Here's how the part is built. I have some questions about the finished solid (model axes, mm). A direction names the side the tool comes from. Give positions to 0.01 mm unless a question says otherwise; leave off trailing zeros. Order: outer loops, then holes, each group sorted by start corner. A loop starts at its lowest first (then second) coordinate and runs counter-clockwise, first axis right, second up. Notation, with made-up numbers: M 57.5,35.5 L 101.5,35.5 A16 cw 101.5,52.5 Z; hole C 44,-6 d8. An arc over 180 degrees is marked long. Use one line per item in the form item = value.
from build123d import *

# Parameters (mm, degrees)
SKETCH1_R           = 14
BOSS_EXTRUDE1_DEPTH = 19
BOSS_EXTRUDE2_DEPTH = 0.8128
SKETCH3_R           = 2.1
CUT_EXTRUDE1_DEPTH  = 0.8128
SKETCH4_R           = 4.5
BOSS_EXTRUDE3_DEPTH = 1.5
BOSS_EXTRUDE4_START = -1.5
SKETCH5_R           = 2.5
BOSS_EXTRUDE4_DEPTH = 10
CUT_EXTRUDE2_DEPTH  = 6
SKETCH7_W           = 14.6
SKETCH7_H           = 5.05387092
BOSS_EXTRUDE5_DEPTH = 16.7


with BuildPart() as part:
    # Sketch1 → Boss-Extrude1 (new body)
    with BuildSketch(Plane(origin=(0, 0, 0), x_dir=(1, 0, 0), z_dir=(0, 1, 0))):
        Circle(SKETCH1_R)
    extrude(amount=-BOSS_EXTRUDE1_DEPTH)

    # Sketch2 → Boss-Extrude2 (add)
    with BuildSketch(Plane(origin=(0, 0, 0), x_dir=(1, 0, 0), z_dir=(0, 1, 0))):
        with BuildLine():
            Line((-17.5, 3.5), (17.5, 3.5))
            ThreePointArc((17.5, 3.5), (21, 0), (17.5, -3.5))
            Line((17.5, -3.5), (-17.5, -3.5))
            ThreePointArc((-17.5, -3.5), (-21, 0), (-17.5, 3.5))
        make_face()
    extrude(amount=-BOSS_EXTRUDE2_DEPTH)

    # Sketch3 → Cut-Extrude1 (cut)
    with BuildSketch(Plane(origin=(0, 0, 0), x_dir=(1, 0, 0), z_dir=(0, 1, 0))):
        with Locations((-17.5, 0)):
            Circle(SKETCH3_R)
        with Locations((17.5, 0)):
            Circle(SKETCH3_R)
    extrude(amount=-CUT_EXTRUDE1_DEPTH, mode=Mode.SUBTRACT)

    # Sketch4 → Boss-Extrude3 (add)
    with BuildSketch(Plane(origin=(0, 0, 0), x_dir=(1, 0, 0), z_dir=(0, 1, 0))):
        with Locations((0, 8)):
            Circle(SKETCH4_R)
    extrude(amount=BOSS_EXTRUDE3_DEPTH)

    # Sketch5 → Boss-Extrude4 (add)
    with BuildSketch(Plane(origin=(0, 1.5, 0), x_dir=(1, 0, 0), z_dir=(0, 1, 0)).offset(BOSS_EXTRUDE4_START)):
        with Locations((0, 8)):
            Circle(SKETCH5_R)
    extrude(amount=BOSS_EXTRUDE4_DEPTH)

    # Sketch6 → Cut-Extrude2 (cut)
    with BuildSketch(Plane(origin=(0, 10, 0), x_dir=(1, 0, 0), z_dir=(0, 1, 0))):
        with BuildLine():
            ThreePointArc((2, 9.5), (0, 10.5), (-2, 9.5))
            Line((-2, 9.5), (2, 9.5))
        make_face()
        with BuildLine():
            Line((2, 6.5), (-2, 6.5))
            ThreePointArc((-2, 6.5), (0, 5.5), (2, 6.5))
        make_face()
    extrude(amount=-CUT_EXTRUDE2_DEPTH, mode=Mode.SUBTRACT)

    # Sketch7 → Boss-Extrude5 (add)
    with BuildSketch(Plane(origin=(0, 0, 0), x_dir=(1, 0, 0), z_dir=(0, 1, 0))):
        with Locations((0, -14.47306454)):
            Rectangle(SKETCH7_W, SKETCH7_H)
    extrude(amount=-BOSS_EXTRUDE5_DEPTH)


solid = part.part
Q1. On a 3-axis mill with a long thin cutter (end or side, diameter ignored), from which of +Z, -Z, +X, -X, +Y, -Y can I reach the whole of each face in a straight line? I mean faces 1 (the face through (0, 7, -6.5)), 2 (the face through (-7.3, -8, 15)), 3 (the face through (0, 7, -9.5)), 4 (the face through (-1.82, -9.37, -13.88)). Say none if no direction works.
Found:
face_1 = +Z, +X, -X, +Y
face_2 = +Z, -X, +Y, -Y
face_3 = -Z, +X, -X, +Y
face_4 = -Y
Q2. I'm going to push flat-ended pins straight in: pin 1 Ø8 at (x, z) = (12.5, -8) entering from +Y; pin 2 Ø2 at (y, z) = (-15.5, -8) entering from -X; pin 3 Ø8 at (x, y) = (5, -13.5) entering from -Z. Where does each tip first touch, or does it pass through?
Found:
pin_1 = 0
pin_2 = -12.12
pin_3 = -13.96
Q3. I want a section at A-A on z = 0. Write out the boundary of the cut face in (x, y).
Found:
outline = M -21,-0.81 L -19.6,-0.81 L -19.6,0 L -21,0 Z; M -15.4,-0.81 L -14,-0.81 L -14,-19 L 14,-19 L 14,-0.81 L 15.4,-0.81 L 15.4,0 L -15.4,0 Z; M 19.6,-0.81 L 21,-0.81 L 21,0 L 19.6,0 Z
Q4. I want a section at C-C on y = 6.25. Write out the boundary of the cut face in (x, z).
Found:
outline = M -2,-9.5 L 2,-9.5 A2.5 ccw 2,-6.5 L -2,-6.5 A2.5 ccw Z
Q5. Thinking about a two-plate mould opening in X: for faces 5 (the face through (-15.497, -0.401, -0.631)), 6 (the face through (16, -0.813, 2)), 7 (the face through (-0.59, 0.74, -12.46)), which applies, +X half, -X half, draft (parallel to the pull), parting line (faces both ways), or undercut?
Found:
face_5 = undercut
face_6 = draft
face_7 = parting line
Q6. I want a section at D-D on z = -8. Write out the boundary of the cut face in (x, y).
Found:
outline = M -11.49,-19 L 11.49,-19 L 11.49,0 L 4.5,0 L 4.5,1.5 L 2.5,1.5 L 2.5,10 L -2.5,10 L -2.5,1.5 L -4.5,1.5 L -4.5,0 L -11.49,0 Z
Q7. I need wall thicknesses on L1, parallel to X at y = -0.4, z = 0; L2, parallel to Z at x = 17.5, y = -0.3; L3, parallel to X at y = -14.75, z = 14. Which ranges of each line are inside material? Lowest first, please.
Found:
L1 = -21 to -19.6, -15.4 to 15.4, 19.6 to 21
L2 = -3.5 to -2.1, 2.1 to 3.5
L3 = -7.3 to 7.3
Q8. I want a section at B-B on x = 0. Write out the boundary of the cut face in (y, z), then the cut area to 3 significant figures.
Found:
outline = M -19,-14 L 0,-14 L 0,-12.5 L 1.5,-12.5 L 1.5,-10.5 L 4,-10.5 L 4,-9.5 L 10,-9.5 L 10,-6.5 L 4,-6.5 L 4,-5.5 L 1.5,-5.5 L 1.5,-3.5 L 0,-3.5 L 0,17 L -16.7,17 L -16.7,14 L -19,14 Z
area = 626 mm²
